Read the model definition and answer for the solid it produces. Units are mm, in the model's axes. Coordinates: 2 decimals unless noted, no trailing zeros. Order: outer loops, then holes, each group sorted by start corner. A loop starts at its lowest first (then second) coordinate and runs counter-clockwise, first axis right, second up. Notation, with made-up numbers: M 58.5,5 L 71.5,5 A4 cw 71.5,10 Z; hole C -6,73 d6. An arc over 180 degrees is marked long. Put each result on its own line as item: value.
from build123d import *

# Parameters (mm, degrees)
SKETCH1_R           = 14.2875
BOSS_EXTRUDE1_DEPTH = 6.35
FILLET1_R           = 10
FILLET2_R           = 4
FILLET3_R           = 4


with BuildPart() as part:
    # Sketch1 → Boss-Extrude1 (new body)
    with BuildSketch(Plane.XY):
        Polygon((0, 27.94), (0, 0), (353.06, 0), (363.06, 10), (381, 27.94), (381, 55.88), (27.94, 55.88), align=None)
        with Locations((38.1, 25.7175)):
            Circle(SKETCH1_R, mode=Mode.SUBTRACT)
        with BuildLine():
            Line((132.645867363, 10), (69.059384531, 10))
            Line((69.059384531, 10), (131.13384809, 35.861727885))
            ThreePointArc((131.13384809, 35.861727885), (128.153903852, 22.712439471), (132.645867363, 10))
        make_face(mode=Mode.SUBTRACT)
        with Locations((152.4, 24.13)):
            Circle(SKETCH1_R, mode=Mode.SUBTRACT)
        with Locations((228.6, 24.13)):
            Circle(SKETCH1_R, mode=Mode.SUBTRACT)
        with BuildLine():
            Line((208.845867363, 10), (172.736964373, 10))
            ThreePointArc((172.736964373, 10), (176.759470296, 28.58704238), (166.416173693, 44.54557971))
            Line((166.416173693, 44.54557971), (215.443755804, 44.54557971))
            ThreePointArc((215.443755804, 44.54557971), (204.743711621, 28.686331972), (208.845867363, 10))
        make_face(mode=Mode.SUBTRACT)
        with BuildLine():
            Line((324.38398396, 10), (262.377905487, 10))
            Line((262.377905487, 10), (321.240476687, 36.706026112))
            ThreePointArc((321.240476687, 36.706026112), (318.779024724, 22.878273345), (324.38398396, 10))
        make_face(mode=Mode.SUBTRACT)
        with Locations((342.9, 25.7175)):
            Circle(SKETCH1_R, mode=Mode.SUBTRACT)
        with BuildLine():
            ThreePointArc((60.896352165, 17.338419846), (61.203129855, 33.209365398), (51.640910235, 45.88))
            Line((51.640910235, 45.88), (125.940457816, 45.88))
            Line((125.940457816, 45.88), (60.896352165, 17.338419846))
        make_face(mode=Mode.SUBTRACT)
        with BuildLine():
            ThreePointArc((251.928870535, 17.373783913), (251.345714342, 32.645581912), (241.756244196, 44.54557971))
            Line((241.756244196, 44.54557971), (317.257409157, 44.54557971))
            Line((317.257409157, 44.54557971), (251.928870535, 17.373783913))
        make_face(mode=Mode.SUBTRACT)
    extrude(amount=BOSS_EXTRUDE1_DEPTH)

    # Fillet1
    fillet1_edges = [part.edges().sort_by_distance(p)[0] for p in [
        (0, 0, 3.175),
        (0, 27.94, 3.175),
        (27.94, 55.88, 3.175),
        (381, 55.88, 3.175),
        (381, 27.94, 3.175),
        (353.06, 0, 3.175),
    ]]
    fillet(fillet1_edges, radius=FILLET1_R)

    # Fillet2
    fillet2_edges = [part.edges().sort_by_distance(p)[0] for p in [
        (208.845867363, 10, 3.175),
        (215.443755804, 44.54557971, 3.175),
        (166.416173693, 44.54557971, 3.175),
        (172.736964373, 10, 3.175),
        (69.059384531, 10, 3.175),
        (131.13384809, 35.861727885, 3.175),
        (125.940457816, 45.88, 3.175),
        (60.896352165, 17.338419846, 3.175),
        (251.928870535, 17.373783913, 3.175),
        (317.257409157, 44.54557971, 3.175),
        (321.240476687, 36.706026112, 3.175),
        (262.377905487, 10, 3.175),
    ]]
    fillet(fillet2_edges, radius=FILLET2_R)

    # Fillet3
    fillet3_edges = [part.edges().sort_by_distance(p)[0] for p in [
        (132.645867363, 10, 3.175),
        (51.640910235, 45.88, 3.175),
        (241.756244196, 44.54557971, 3.175),
        (324.38398396, 10, 3.175),
    ]]
    fillet(fillet3_edges, radius=FILLET3_R)


solid = part.part
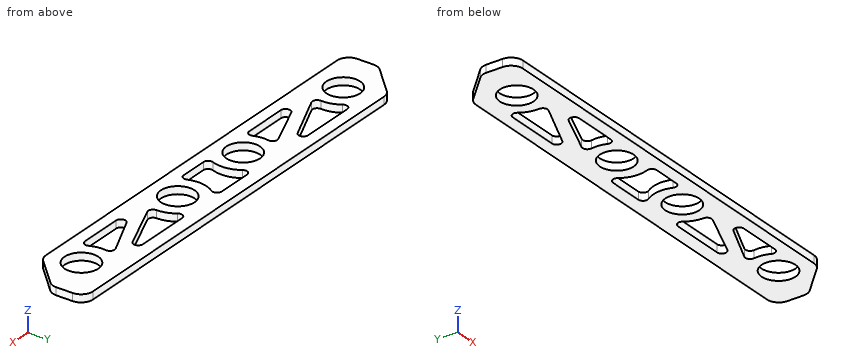
Q1. Consider line 1 along Y through (x, z) = (199.5, 4.75); line 2 along Y through (x, z) = (342.9, 5.25) (3 decimals); line 3 along Y through (x, z) = (102, 1.5). Determine where each line is inside the solid, lowest interval first.
Answers below:
line 1: y = 0 to 10, 44.55 to 55.88
line 2: y = 0 to 11.43, 40.005 to 55.88
line 3: y = 0 to 10, 23.72 to 35.37, 45.88 to 55.88
Q2. Find section A-A on x = 152.4. Write down the section's boundary in (y, z).
Answers below:
outline: M 0,0 L 9.84,0 L 9.84,6.35 L 0,6.35 Z; M 38.42,0 L 55.88,0 L 55.88,6.35 L 38.42,6.35 Z
Q3. Find section B-B on z = 1.75. Give the number of separate pieces and of enclosed holes in the cut face, plus the area to 3 significant figures.
Answers below:
separate pieces: 1
enclosed holes: 9
area: 13,800 mm^2
